CAD build for the part. Positions are in the model's coordinates, mm. A direction names the side the tool comes from. Coordinates: 2 decimals unless noted, no trailing zeros. Order: outer loops, then holes, each group sorted by start corner. A loop starts at its lowest first (then second) coordinate and runs counter-clockwise, first axis right, second up. Notation, with made-up numbers: (-9, -0.75) - (19, -0.75) arc R20 ccw to (19, 15.25) - close; hole circle Ø11 at (81, 3). An arc over 180 degrees is marked (long way). Write each question's results on one line, items separated by ' | '. Start each with the question number.
Q1. Pull direction Y, two halves, no side cores. Call faces 6 (the cylindrical face through (10.18, -11.457, 9.569)), 7 (the flat face through (3, -9, 0)), 8 (the flat face through (23, 0, 13)), 9 (the cylindrical face through (25.403, -15.735, 12.789)): released by +Y, released by -Y, zero draft, split by the parting line, or undercut.
Q2. Pin check, flat tips, straight feed: P1, Ø10, axis at x = 12.7, y = -9.525, coming from the -Z side; P2, Ø1.9, axis at y = -11.5, z = 4.5, coming from the +X side; P3, Ø3, axis at x = 32.5, z = 23, coming from the -Y side. Stop position of each tip, or through.
Q3. Band-saw the part on C-C, the plane y = -4. Write the cut outline in (x, z).
Q4. Which spindle directions (+Z, -Z, +X, -X, +Y, -Y) get a long thin tool onto all of the face, cutting with end or side? Do faces 1 (the flat face through (3, -19.05, 3)), 2 (the flat face through (38.1, -13, 14)), 3 (the flat face through (10, -13, 12.7)), 4 (the flat face through (33, -16, 19.05)), 5 (the flat face through (6.35, -9, 3)). Say none if no direction does.
Q5. Band-saw the part on B-B, the plane y = -10.5. Write the cut outline in (x, z), then the cut area to 3 significant figures.
Q6. Wall check: probe 1 along Y at (x, z) = (12.5, 10); probe 2 along Z at (x, y) = (25, -21.25); probe 3 along Z at (x, y) = (32, -5.5). Give the ranges that are in metal, low to high.
Q7. Band-saw the part on A-A, the plane x = 12.7. Write the cut outline in (y, z).
Q8. Band-saw the part on D-D, the plane z = 2.5. Write the cut outline in (x, y).
```python
from build123d import *

# Parameters (mm, degrees)
F0_W     = 6.35
F0_H     = 6.35
F1_DEPTH = 19.05
F2_DEPTH = 25.4
F0_W_2   = 19.05
F3_DEPTH = 6.35
F4_R     = 3.175
F5_DEPTH = 25.4
F6_R     = 3.175
F7_DEPTH = 25.4


with BuildPart() as f1:
    # F0 (on Front) → F1 (new body)
    with BuildSketch(Plane.XZ):
        with Locations((3.175, 3.175)):
            Rectangle(F0_W, F0_H)
    extrude(amount=F1_DEPTH)

    # F0 (on Front) → F2 (join)
    with BuildSketch(Plane.XZ):
        Polygon((0, 12.7), (0, 6.35), (6.35, 6.35), (38.1, 6.35), (38.1, 19.05), (19.05, 19.05), (19.05, 12.7), align=None)
    extrude(amount=F2_DEPTH)

    # F0 (on Front) → F3 (join)
    with BuildSketch(Plane.XZ):
        with Locations((28.575, 22.225)):
            Rectangle(F0_W_2, F0_H)
    extrude(amount=F3_DEPTH)

    # F4 (on face) → F5 (cut)
    with BuildSketch(Plane.XY.offset(12.7)):
        with Locations((12.7, -9.525)):
            Circle(F4_R)
    extrude(amount=-F5_DEPTH, mode=Mode.SUBTRACT)

    # F6 (on face) → F7 (cut)
    with BuildSketch(Plane.XY.offset(19.05)):
        with Locations((28.575, -15.875)):
            Circle(F6_R)
    extrude(amount=-F7_DEPTH, mode=Mode.SUBTRACT)


solid = f1.part
```
Results below:
1) face 6: undercut | face 7: zero draft | face 8: released by +Y | face 9: undercut
2) P1: stops at z = 6.35 | P2: stops at x = 6.35 | P3: stops at y = -6.35
3) outline: (0, 0) - (6.35, 0) - (6.35, 6.35) - (38.1, 6.35) - (38.1, 25.4) - (19.05, 25.4) - (19.05, 12.7) - (0, 12.7) - close
4) face 1: -Z, +X, -X, -Y | face 2: +Z, -Z, +X, +Y, -Y | face 3: +Z, -X, +Y, -Y | face 4: +Z, +X, -X, -Y | face 5: -Z, +X, +Y, -Y
5) outline: (0, 0) - (6.35, 0) - (6.35, 6.35) - (9.68, 6.35) - (9.68, 12.7) - (0, 12.7) - close; (15.72, 6.35) - (38.1, 6.35) - (38.1, 19.05) - (19.05, 19.05) - (19.05, 12.7) - (15.72, 12.7) - close | area: 365 mm²
6) probe 1: y = -25.4 to -12.69, -6.36 to 0 | probe 2: z = 6.35 to 19.05 | probe 3: z = 6.35 to 25.4
7) outline: (-25.4, 6.35) - (-12.7, 6.35) - (-12.7, 12.7) - (-25.4, 12.7) - close; (-6.35, 6.35) - (0, 6.35) - (0, 12.7) - (-6.35, 12.7) - close
8) outline: (0, -19.05) - (6.35, -19.05) - (6.35, 0) - (0, 0) - close
